For this review, take the finished solid that the model builds, in its own axes (mm). Coordinates: 2 decimals unless noted, no trailing zeros. Write each loop counter-clockwise with the first axis right and the second up, starting at its lowest first coordinate (ties: lowest second). Pieces come first, ordered by that corner, then holes.
```python
from build123d import *

# Parameters (mm, degrees)
F0_R     = 2.5
F1_DEPTH = 3.5
F2_W     = 2.3748684174
F2_H     = 0.3
F3_DEPTH = 7.001
F4_R     = 2
F5_DEPTH = 3
F7_R     = 1


# Not quite as in the source:
# - a pattern or mirror of a feature is missing from the dataset's text; its kind, count and spacing are read off the source's solid


with BuildPart() as f1:
    # F0 (on Front) → F1 (new body, symmetric)
    with BuildSketch(Plane.XZ):
        Circle(F0_R)
    extrude(amount=F1_DEPTH, both=True)

    # F2 (on face) → F3 (cut, through all)
    with BuildSketch(Plane.XZ.offset(3.5)):
        with Locations((0, 2.35)):
            Rectangle(F2_W, F2_H)
    extrude(amount=-F3_DEPTH, mode=Mode.SUBTRACT)

    # F4 (on face) → F5 (join)
    with BuildSketch(Plane.XZ.offset(3.5)):
        Circle(F4_R)
    f5 = extrude(amount=F5_DEPTH)

    # F5_copies: F5 across plane
    add(f5.mirror(Plane.ZX))

    # F8: sweep along a path in F6
    with BuildLine(Plane.XY) as f8_path:
        Line((0, 7), (0, -7))
        ThreePointArc((0, -7), (0.1882968799, -8.2128146291), (0.7354596623, -9.3114446529))
        ThreePointArc((0.7354596623, -9.3114446529), (30, 0), (0.7354596623, 9.3114446529))
        ThreePointArc((0.7354596623, 9.3114446529), (0.1882968799, 8.2128146291), (0, 7))
    # F7 (on face) → F8 (sweep)
    with BuildSketch(Plane.XZ.offset(6.5)):
        Circle(F7_R)
    sweep(path=f8_path.line)


solid = f1.part
```
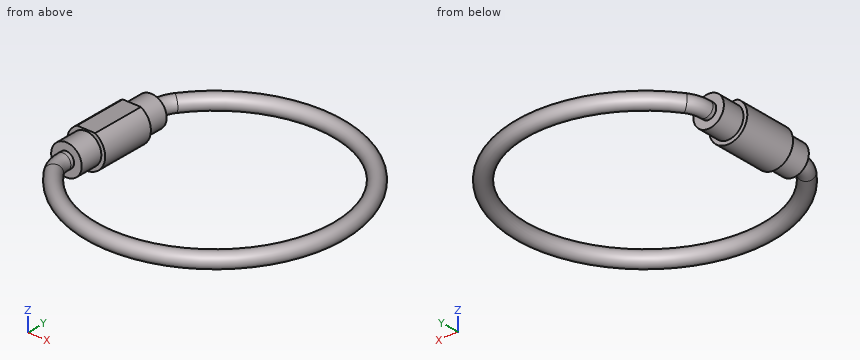
Q1. For probe 1 along Y at (x, z) = (19, 0.25); probe 2 along Y at (x, z) = (-0.5, 1.6); probe 3 along Y at (x, z) = (6, 0.35), list the stretches that pass through material, from the lowest coordinate up.
Ans:
probe 1: y = -16.3 to -14.26, 14.26 to 16.3
probe 2: y = -6.5 to 6.5
probe 3: y = -15.12 to -12.97, 12.97 to 15.12
Q2. Add section A-A (z = 0). State the section outline as (x, y) points, then the cut area to 3 significant figures.
Ans:
outline: (-2.5, -3.5) - (-2, -3.5) - (-2, -6.5) - (-1, -6.5) - (-1, -7) arc R5 ccw to (-0.08, -9.89) arc R17.11 ccw (long way) to (-0.08, 9.89) arc R5 ccw to (-1, 7) - (-1, 6.5) - (-2, 6.5) - (-2, 3.5) - (-2.5, 3.5) - close; hole (1, -7) arc R3 ccw to (1.55, -8.73) arc R15.11 ccw (long way) to (1.55, 8.73) arc R3 ccw to (1, 7) - (1, 6.5) - (2, 6.5) - (2, 3.5) - (2.5, 3.5) - (2.5, -3.5) - (2, -3.5) - (2, -6.5) - (1, -6.5) - close
area: 234 mm2
Q3. Clearance check with flat-ended pins moving along their axes: pin 1 Ø2.5 at (x, z) = (1, 0.5) entering from +Y; pin 2 Ø1.2 at (x, z) = (-1, 0.5) entering from +Y; pin 3 Ø2 at (x, z) = (0, -1) entering from -Y. State where each tip first meets the part, or that it passes through.
Ans:
pin 1: stops at y = 12.49
pin 2: stops at y = 9.21
pin 3: stops at y = -10.9
